```python
from build123d import *

# Parameters (mm, degrees)
SKETCH1_R           = 25.4
SKETCH1_R_2         = 22.225
BOSS_EXTRUDE1_DEPTH = 914.4
CUT_EXTRUDE1_START  = -100.0125
SKETCH2_R           = 25.4
CUT_EXTRUDE1_DEPTH  = 816.09278356
CUT_EXTRUDE3_DEPTH  = 107.267681617
SKETCH6_R           = 15.875
CUT_EXTRUDE5_DEPTH  = 107.267681617


with BuildPart() as part:
    # Sketch1 → Boss-Extrude1 (new body)
    with BuildSketch(Plane.XY):
        Circle(SKETCH1_R)
        Circle(SKETCH1_R_2, mode=Mode.SUBTRACT)
    extrude(amount=BOSS_EXTRUDE1_DEPTH)

    # Sketch2 → Cut-Extrude1 (cut, through all)
    with BuildSketch(Plane(origin=(0, 0, 0), x_dir=(-1, 0, 0), z_dir=(0, 0, -1)).offset(CUT_EXTRUDE1_START)):
        Circle(SKETCH2_R)
    extrude(amount=-CUT_EXTRUDE1_DEPTH, mode=Mode.SUBTRACT)

    # Sketch4 → Cut-Extrude3 (cut, through all)
    with BuildSketch(Plane.XY):
        with BuildLine():
            Line((-25.4, 0), (25.4, 0))
            ThreePointArc((25.4, 0), (0, 25.4), (-25.4, 0))
        make_face()
    extrude(amount=CUT_EXTRUDE3_DEPTH, mode=Mode.SUBTRACT)

    # Sketch6 → Cut-Extrude5 (cut, through all)
    with BuildSketch(Plane(origin=(0, 0, 0), x_dir=(1, 0, 0), z_dir=(0, 1, 0))):
        with Locations(Location((0, -77.121807345, 0), (0, 0, 270))):
            Circle(SKETCH6_R)
    extrude(amount=-CUT_EXTRUDE5_DEPTH, mode=Mode.SUBTRACT)


solid = part.part
```
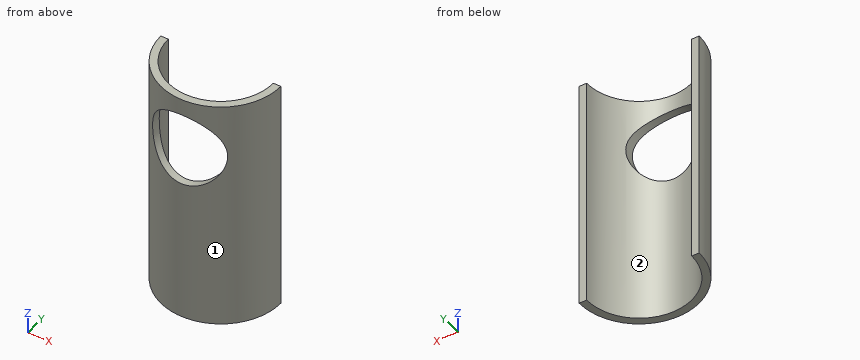
Input: part model. Units: mm. Frame: model coordinates. Face numbers are marked on the shaded views. Coordinates: 2 decimals unless noted, no trailing zeros. Loops run counter-clockwise (first coordinate to the right, second up) from the corner with the lowest first, then second, coordinate; pieces in that order, holes last. Notation, with made-up numbers: M 50.5,68 L 85.5,68 A24 ccw 85.5,103 Z; hole C -6,19 d8. An arc over 180 degrees is marked long. Use a Markdown table: item, result. Add a question column.
1) Pin query (flat end, axial travel): P1, Ø1.5, axis at y = -7, z = 40.5, coming from the -X side; P2, Ø1, axis at x = 18.5, z = 63.5, coming from the +Y side; P3, Ø5, axis at y = -17, z = 34, coming from the -X side. Return the tip coordinate at first contact, or that it passes through.
2) Section C-C, the plane z = 39. Return the cut outline in (x, y) (3 decimals).
3) Section A-A, the plane x = 0. Return the cut outline in (y, z) (1 decimal).
4) Draft query along X for the marked faces 1 and 2. Return one class per face: +X half, -X half, draft (parallel to the pull), parting line (faces both ways), or undercut.
5) Line query: L1, parallel to X at y = -12.5, z = 20.5; L2, parallel to X at y = -10.5, z = 24; L3, parallel to Z at x = 7.5, y = -21.75. Output: solid intervals per line, ascending. Write a range as from..to.
6) Section B-B, the plane y = -9. Return the cut outline in (x, z), plus the area to 3 significant figures.
Answer below:
| question | item | result |
|---|---|---|
| 1 | P1 | x = -24.62 |
| 1 | P2 | y = -11.53 |
| 1 | P3 | x = -20.85 |
| 2 | outline | M -25.4,0 A25.4 ccw 25.4,0 L 22.225,0 A22.225 cw -22.225,0 Z |
| 3 | outline | M -25.4,0 L -22.2,0 L -22.2,61.2 L -25.4,61.2 Z; M -25.4,93 L -22.2,93 L -22.2,100 L -25.4,100 Z |
| 4 | face 1 | parting line |
| 4 | face 2 | undercut |
| 5 | L1 | -22.11..-18.38, 18.38..22.11 |
| 5 | L2 | -23.13..-19.59, 19.59..23.13 |
| 5 | L3 | 0..63.13, 91.11..100.01 |
| 6 | outline | M -23.75,0 L -20.32,0 L -20.32,100.01 L -23.75,100.01 Z; M 20.32,0 L 23.75,0 L 23.75,100.01 L 20.32,100.01 Z |
| 6 | area | 686 mm2 |
